Could you check a few things on this model? Use its own coordinates, in mm. Give positions to 0.01 mm unless a question says otherwise; leave off trailing zeros. Order: outer loops, then holes, each group sorted by start corner. A loop starts at its lowest first (then second) coordinate and runs counter-clockwise, first axis right, second up. Notation, with made-up numbers: (-11, -22) - (1, -22) arc R30 cw to (1, 17) - close; hole circle Ø6 at (34, 56.5). An arc over 180 degrees is marked (long way). Put each result on its own line as item: value.
from build123d import *

# Parameters (mm, degrees)
F0_R     = 1.7
F0_R_2   = 1.5
F1_DEPTH = 2


with BuildPart() as f1:
    # F0 (on Top) → F1 (new body)
    with BuildSketch(Plane.XY):
        Polygon((41.421356, 100), (-41.421356, 100), (-100, 41.421356), (-100, -41.421356), (-41.421356, -100), (41.421356, -100), (102.809891, -49.384143), (202.809891, -49.384143), (202.809891, 33.458857), (102.809891, 33.458857), align=None)
        with Locations((-31.066017, -75)):
            Circle(F0_R, mode=Mode.SUBTRACT)
        with Locations((31.066017, -75)):
            Circle(F0_R, mode=Mode.SUBTRACT)
        with Locations((-75, -31.066017)):
            Circle(F0_R_2, mode=Mode.SUBTRACT)
        with Locations((75, -31.066017)):
            Circle(F0_R, mode=Mode.SUBTRACT)
        with Locations((-75, 31.066017)):
            Circle(F0_R, mode=Mode.SUBTRACT)
        with Locations((-31.066017, 75)):
            Circle(F0_R, mode=Mode.SUBTRACT)
        with Locations((31.066017, 75)):
            Circle(F0_R, mode=Mode.SUBTRACT)
        with Locations((75, 31.066017)):
            Circle(F0_R, mode=Mode.SUBTRACT)
    extrude(amount=F1_DEPTH)


solid = f1.part
1) If I drill on line 1 (X direction, y = -75, z = 1.2); line 2 (Y direction, x = 75, z = 1.5); line 3 (Y direction, x = -75, z = 1.15), over which ranges is the centre line in solid material (lowest first)? Write a range as [from, to].
Filled in:
line 1: x = [-66.42, -32.77], [-29.37, 29.37], [32.77, 71.74]
line 2: y = [-72.31, -32.77], [-29.37, 29.37], [32.77, 63.6]
line 3: y = [-66.42, -32.57], [-29.57, 29.37], [32.77, 66.42]
2) Suppose I cut it at A-A, the plane z = 1.7. State how many separate pieces and enclosed holes the cut face has, and give its area (3 significant figures).
Filled in:
separate pieces: 1
enclosed holes: 8
area: 41,700 mm^2
3) I'm going to push a flat-ended pin straight in: pin 1 (2.5 mm diameter, centred on x = 31.07, y = -75, fed in from +Z). Where does the tip first touch, or does it pass through?
Filled in:
pin 1: passes through
4) Suppose I cut it at B-B, the plane x = 183. List the corners of the cut face in (y, z) for me.
Filled in:
outline: (-49.38, 0) - (33.46, 0) - (33.46, 2) - (-49.38, 2) - close
5) Suppose I cut it at C-C, the plane y = -83. List the corners of the cut face in (x, z) for me.
Filled in:
outline: (-58.42, 0) - (62.04, 0) - (62.04, 2) - (-58.42, 2) - close
